Here's how the part is built. I have some questions about the finished solid (model axes, mm). A direction names the side the tool comes from. Give positions to 0.01 mm unless a question says otherwise; leave off trailing zeros. Write each loop counter-clockwise with the first axis right and the second up, starting at its lowest first coordinate (ties: lowest second). Pieces come first, ordered by that corner, then holes. Notation, with made-up numbers: (23, 86.5) -> (29, 86.5) arc R26 ccw to (29, 113.5) -> close; hole circle Ø8 at (-0.5, -20.75). An arc over 180 degrees is marked (long way). Use one line per item in the form item = value.
```python
from build123d import *

# Parameters (mm, degrees)
F0_W     = 76.2
F0_H     = 19.05
F1_DEPTH = 25.4


with BuildPart() as f1:
    # F0 (on Front) → F1 (new body)
    with BuildSketch(Plane.XZ):
        Polygon((188.914097, 172.629672), (-319.085903, 172.629672), (-319.085903, -189.320328), (-242.885903, -189.320328), (112.714097, -189.320328), (188.914097, -189.320328), align=None)
        Polygon((-166.066591, -99.527862), (-151.572697, -111.890287), (-184.539165, -150.540669), (-199.033058, -138.178244), align=None, mode=Mode.SUBTRACT)
        Polygon((2.964357, 98.646563), (35.930825, 137.296945), (50.424718, 124.93452), (17.458251, 86.284138), align=None, mode=Mode.SUBTRACT)
        with Locations((-280.985903, -198.845328)):
            Rectangle(F0_W, F0_H)
        with Locations((150.814097, -198.845328)):
            Rectangle(F0_W, F0_H)
    extrude(amount=F1_DEPTH)


solid = f1.part
```
Q1. I want a section at A-A, the plane y = -16. Write out the boundary of the cut face in (x, z), and give its area (3 significant figures).
Result set:
outline = (-319.09, -208.37) -> (-242.89, -208.37) -> (-242.89, -189.32) -> (112.71, -189.32) -> (112.71, -208.37) -> (188.91, -208.37) -> (188.91, 172.63) -> (-319.09, 172.63) -> close; hole (-199.03, -138.18) -> (-184.54, -150.54) -> (-151.57, -111.89) -> (-166.07, -99.53) -> close; hole (2.96, 98.65) -> (17.46, 86.28) -> (50.42, 124.93) -> (35.93, 137.3) -> close
area = 185,000 mm2
Q2. Will this pin go through, and if not, where does the flat tip stop? pin 1 Ø12 at (x, y) = (-71, -18.5) entering from -Z.
Result set:
pin_1 = -189.32
Q3. I want a section at D-D, the plane x = -141. Write out the boundary of the cut face in (y, z), and give its area (3 significant figures).
Result set:
outline = (-25.4, -189.32) -> (0, -189.32) -> (0, 172.63) -> (-25.4, 172.63) -> close
area = 9,190 mm2
Q4. If we mould it in two halves opening along X, with no side actions, what happens to faces 4 (the face through (-69, 0, -15)), 5 (the face through (112.714, -13, -199)), 6 (the face through (-319.086, -13, -15))? For each: +X half, -X half, draft (parallel to the pull), parting line (faces both ways), or undercut.
Result set:
face_4 = draft
face_5 = undercut
face_6 = -X half
Q5. I want a section at C-C, the plane z = 115.5. Write out the boundary of the cut face in (x, y), and give its area (3 significant figures).
Result set:
outline = (-319.09, -25.4) -> (17.34, -25.4) -> (17.34, 0) -> (-319.09, 0) -> close; (42.38, -25.4) -> (188.91, -25.4) -> (188.91, 0) -> (42.38, 0) -> close
area = 12,300 mm2
Q6. If I drill on line 1 along X through (y, z) = (-16.25, -192); line 2 along Z through (x, y) = (75, -21.5); line 3 along X through (y, z) = (-15.75, 135), over which ranges is the centre line in solid material (lowest first)? Write a range as from..to.
Result set:
line_1 = -319.09..-242.89, 112.71..188.91
line_2 = -189.32..172.63
line_3 = -319.09..33.97, 38.62..188.91
Q7. I want a section at B-B, the plane x = 25. Write out the boundary of the cut face in (y, z), and give its area (3 significant figures).
Result set:
outline = (-25.4, -189.32) -> (0, -189.32) -> (0, 95.13) -> (-25.4, 95.13) -> close; (-25.4, 124.48) -> (0, 124.48) -> (0, 172.63) -> (-25.4, 172.63) -> close
area = 8,450 mm2
Q8. Which directions (+Z, -Z, +X, -X, +Y, -Y) give clear straight access to the entire face, cutting with the end or side of a thin tool? Please do faces 1 (the face through (-182.78, -12.52, -119.12)), 2 (the face through (-242.886, -13, -199)), 3 (the face through (-282, -13, -208.37)).
Result set:
face_1 = +Y, -Y
face_2 = -Z, +Y, -Y
face_3 = -Z, +X, -X, +Y, -Y
